For this review, use the dimensioned drawing (mm, ordinates from the lowest corner) and the shaded views. Coordinates: 2 decimals unless noted, no trailing zeros. Write each loop counter-clockwise with the first axis right and the second up, starting at its lowest first coordinate (ties: lowest second). Pieces come first, ordered by that corner, then holes. Notation, with made-up numbers: (71.5, -18.75) - (103.5, -18.75) arc R11 ccw to (103.5, -8.75) - close; hole circle Ø11 at (85.5, -22). An arc over 180 degrees is marked (long way). Put each result on its own line as item: value.
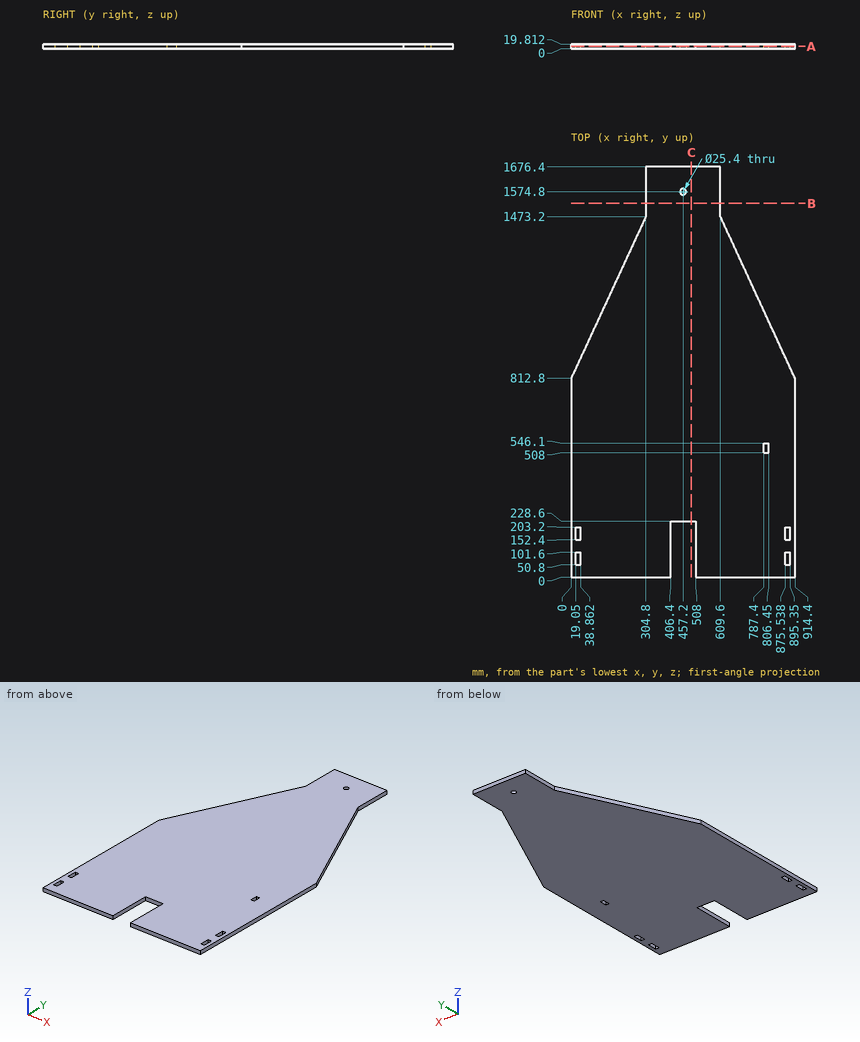
1. Consider section C-C on x = 491. State the section outline as (y, z) points.
Determined:
outline: (228.6, 0) - (1676.4, 0) - (1676.4, 19.81) - (228.6, 19.81) - close
2. Consider section B-B on y = 1527. State the section outline as (x, z) points, plus the area to 3 significant figures.
Determined:
outline: (304.8, 0) - (609.6, 0) - (609.6, 19.81) - (304.8, 19.81) - close
area: 6,040 mm^2
3. For pin 1 Ø5 at (y, z) = (1015, 16.5) entering from -X; pin 2 Ø23 at (x, y) = (457.2, 1574.8) entering from -Z; pin 3 Ø10 at (x, z) = (883.5, 11.5) entering from +Y; pin 4 Ø1.5 at (y, z) = (1246, 12.5) entering from -X, all flat-tipped, find the tip position at first contact; note any pin that passes through.
Determined:
pin 1: stops at x = 92.17
pin 2: passes through
pin 3: stops at y = 890.58
pin 4: stops at x = 199.59
4. To check wall thickness, follow probe 1 along Y at (x, z) = (457.2, 14.5); probe 2 along X at (y, z) = (1574.8, 14); probe 3 along Y at (x, z) = (437, 8). State the ranges of each line that lie inside material, in increasing order.
Determined:
probe 1: y = 228.6 to 1562.1, 1587.5 to 1676.4
probe 2: x = 304.8 to 444.5, 469.9 to 609.6
probe 3: y = 228.6 to 1676.4
5. Consider section A-A on z = 10.25. Give the number of separate pieces and of enclosed holes in the cut face, plus the area to 3 significant figures.
Determined:
separate pieces: 1
enclosed holes: 6
area: 1,180,000 mm^2
